Design review of the part shown in the three views and the two pictorial views. Dimensions are in mm from the part's minimum x, y and z. A direction names the side the tool comes from. Give positions to 0.01 mm unless a question says otherwise; leave off trailing zeros. Write each loop counter-clockwise with the first axis right and the second up, starting at its lowest first coordinate (ties: lowest second). Pieces come first, ordered by that corner, then holes. Notation, with made-up numbers: M 25,69 L 35,69 A15 ccw 35,92 Z; hole C -24,41.5 d9. An arc over 180 degrees is marked long. Write item = value, one per line.
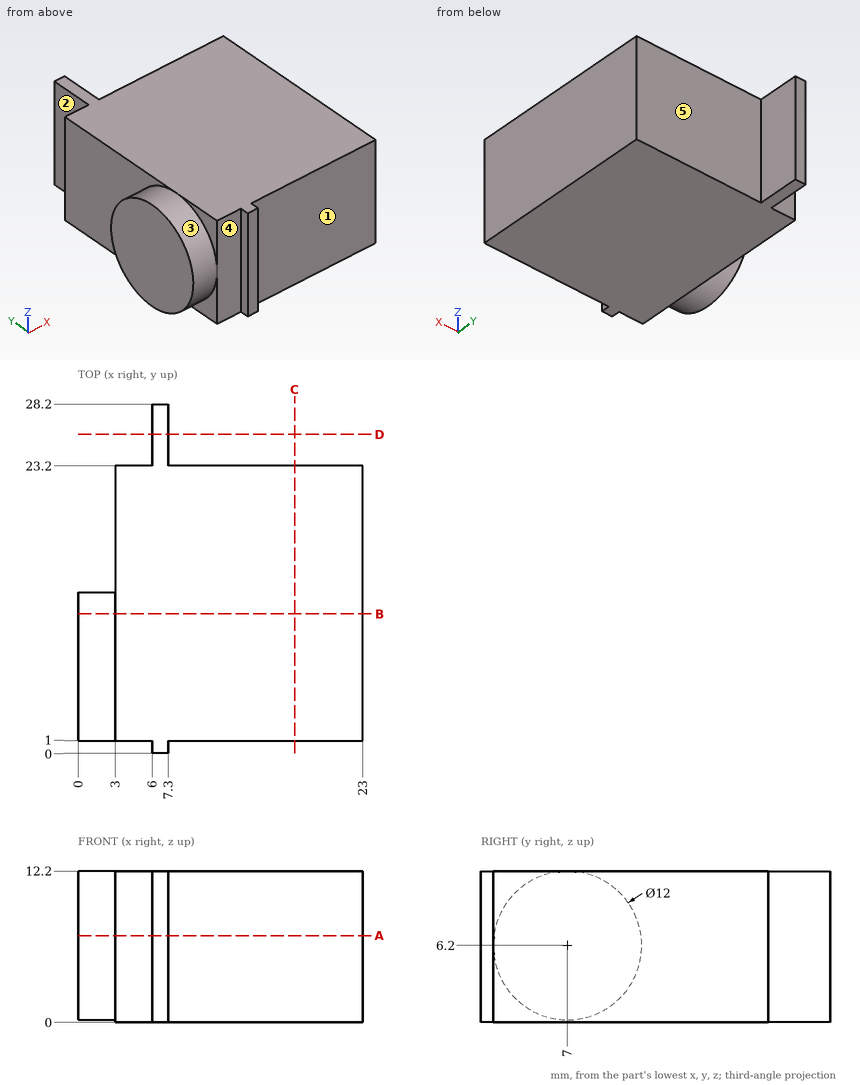
1. We need section B-B, the plane y = 11.25. Write out the cut boundary in (x, z), then the cut area to 3 significant figures.
Responses:
outline = M 0,1.96 L 3,1.96 L 3,0 L 23,0 L 23,12.2 L 3,12.2 L 3,10.44 L 0,10.44 Z
area = 269 mm2
2. Insertion check: P1, Ø2, axis at x = 9, z = 6, coming from the -Y side; P2, Ø6, axis at x = 10.5, y = 4.5, coming from the -Z side; P3, Ø0.8, axis at y = 0.5, z = 3.5, coming from the +X side; P4, Ø5, axis at y = 19.5, z = 8.5, coming from the -X side. Each pin has a flat end and moves straight along its axis. Give the tip position at first contact, or say it passes through.
Responses:
P1 = 1
P2 = 0
P3 = 7.3
P4 = 3
3. We need section D-D, the plane y = 25.75. Write out the cut boundary in (x, z).
Responses:
outline = M 6,0 L 7.3,0 L 7.3,12.2 L 6,12.2 Z
4. We need section A-A, the plane z = 7. Write out the cut boundary in (x, y), then the cut area to 3 significant figures.
Responses:
outline = M 0,1.05 L 3,1.05 L 3,1 L 6,1 L 6,0 L 7.3,0 L 7.3,1 L 23,1 L 23,23.2 L 7.3,23.2 L 7.3,28.2 L 6,28.2 L 6,23.2 L 3,23.2 L 3,12.95 L 0,12.95 Z
area = 487 mm2
5. Machinability: for the marked faces 1, 2, 3, 4 and 5, which of the approach directions +Z, -Z, +X, -X, +Y, -Y give a long, thin tool a straight path to every point of the face, cutting with its end or side? Answer none if there is none.
Responses:
face_1 = +Z, -Z, +X, -Y
face_2 = +Z, -Z, -X, +Y
face_3 = -X
face_4 = +Z, -Z, -X, -Y
face_5 = +Z, -Z, +X, +Y
6. We need section C-C, the plane x = 17.5. Write out the cut boundary in (y, z), then the cut area to 3 significant figures.
Responses:
outline = M 1,0 L 23.2,0 L 23.2,12.2 L 1,12.2 Z
area = 271 mm2
7. For line 1 along Y through (x, z) = (9, 4.5); line 2 along X through (y, z) = (11, 11.25); line 3 along X through (y, z) = (23.75, 2), list the stretches that pass through material, from the lowest coordinate up. Write a range as from..to.
Responses:
line_1 = 1..23.2
line_2 = 3..23
line_3 = 6..7.3
